```python
from build123d import *

# Parameters (mm, degrees)
ESQUISSE2_W             = 110
ESQUISSE2_H             = 106
BOSS_EXTRU_3_DEPTH      = 5
BOSS_EXTRU_4_DEPTH      = 3
BOSS_EXTRU_5_DEPTH      = 2
BOSS_EXTRU_6_DEPTH      = 5.5
BOSS_EXTRU_7_DEPTH      = 110
ESQUISSE7_R             = 2.35
ENL_V_MAT_EXTRU_1_DEPTH = 12
CONG_3_R                = 8
ENL_V_MAT_EXTRU_2_DEPTH = 4
CHANFREIN1_SIZE         = 0.5


with BuildPart() as part:
    # Esquisse2 → Boss.-Extru.3 (new body)
    with BuildSketch(Plane(origin=(0, 0, 0), x_dir=(1, 0, 0), z_dir=(0, 1, 0))):
        with Locations((55, 53)):
            Rectangle(ESQUISSE2_W, ESQUISSE2_H)
    extrude(amount=BOSS_EXTRU_3_DEPTH)

    # Esquisse3 → Boss.-Extru.4 (add)
    with BuildSketch(Plane(origin=(0, 5, 0), x_dir=(1, 0, 0), z_dir=(0, 1, 0))):
        Polygon((7, 4), (7, 106), (0, 106), (0, 0), (110, 0), (110, 106), (103, 106), (103, 4), align=None)
    extrude(amount=BOSS_EXTRU_4_DEPTH)

    # Esquisse4 → Boss.-Extru.5 (add)
    with BuildSketch(Plane(origin=(0, 8, 0), x_dir=(1, 0, 0), z_dir=(0, 1, 0))):
        Polygon((4, 106), (4, 4), (106, 4), (106, 106), (110, 106), (110, 0), (0, 0), (0, 106), align=None)
    extrude(amount=BOSS_EXTRU_5_DEPTH)

    # Esquisse6 → Boss.-Extru.6 (add)
    with BuildSketch(Plane(origin=(0, 10, 0), x_dir=(1, 0, 0), z_dir=(0, 1, 0))):
        Polygon((0, 106), (7, 106), (7, 4), (103, 4), (103, 106), (110, 106), (110, 4), (110, 0), (0, 0), (0, 4), align=None)
    extrude(amount=BOSS_EXTRU_6_DEPTH)

    # Esquisse8 → Boss.-Extru.7 (add)
    with BuildSketch(Plane(origin=(110, 0, 0), x_dir=(0, 0, -1), z_dir=(1, 0, 0))):
        Polygon((0, 0), (106, 0), (106, -18.690659955), align=None)
    extrude(amount=-BOSS_EXTRU_7_DEPTH)

    # Esquisse7 → Enlèv. mat.-Extru.1 (cut)
    with BuildSketch(Plane(origin=(0, 0, -106), x_dir=(-1, 0, 0), z_dir=(0, 0, -1))):
        with Locations((-103, 0)):
            Circle(ESQUISSE7_R)
        with Locations((-7, 0)):
            Circle(ESQUISSE7_R)
    extrude(amount=-ENL_V_MAT_EXTRU_1_DEPTH, mode=Mode.SUBTRACT)

    # Congé3
    cong_3_edges = [part.edges().sort_by_distance(p)[0] for p in [
        (110, 7.75, 0),
        (0, 7.75, 0),
    ]]
    fillet(cong_3_edges, radius=CONG_3_R)

    # Esquisse9 → Enlèv. mat.-Extru.2 (cut)
    with BuildSketch(Plane(origin=(0, 0, 0), x_dir=(1, 0, 0), z_dir=(0, -0.9848077530122092, 0.17364817766692348))):
        with BuildLine():
            Line((14, -8), (96, -8))
            ThreePointArc((96, -8), (100.242640687, -9.757359313), (102, -14))
            Line((102, -14), (102, -97.63522086))
            ThreePointArc((102, -97.63522086), (100.242640687, -101.877861547), (96, -103.63522086))
            Line((96, -103.63522086), (14, -103.63522086))
            ThreePointArc((14, -103.63522086), (9.757359313, -101.877861547), (8, -97.63522086))
            Line((8, -97.63522086), (8, -14))
            ThreePointArc((8, -14), (9.757359313, -9.757359313), (14, -8))
        make_face()
    extrude(amount=-ENL_V_MAT_EXTRU_2_DEPTH, mode=Mode.SUBTRACT)

    # Chanfrein1
    chanfrein1_edges = [part.edges().sort_by_distance(p)[0] for p in [
        (105.35, 0, -106),
        (9.35, 0, -106),
    ]]
    chamfer(chanfrein1_edges, length=CHANFREIN1_SIZE)


solid = part.part
```
Work out the finished part from the listing and answer in its coordinate system (mm). A direction names the side the tool comes from. Coordinates: 2 decimals unless noted, no trailing zeros. Order: outer loops, then holes, each group sorted by start corner. A loop starts at its lowest first (then second) coordinate and runs counter-clockwise, first axis right, second up. Notation, with made-up numbers: M 67.5,-28.75 L 111.5,-28.75 A19 cw 111.5,-21.75 Z; hole C 75,62.25 d4. An arc over 180 degrees is marked long. Use CSV: the item, a comma, the result in double quotes.
1) For faces 5 (the face through (7, 6, -54)), 6 (the face through (105, 10, -56)), 7 (the face through (100.2, 0.26, -9.91)), determine the directions among +Z, -Z, +X, -X, +Y, -Y from which every point of the face is accessible in a straight line to the end or side of a thin tool.
Worked out:
face 5,"-Z, +Y"
face 6,"-Z"
face 7,"-Y"
2) Section D-D on z = -98.5 is taken. Count the separate pieces of the cut face and the enclosed holes in it, plus the area to 3 significant figures.
Worked out:
separate pieces,"1"
enclosed holes,"2"
area,"2,180 mm^2"
3) Section B-B on z = -27.5 is taken. Write down the section's boundary in (x, y).
Worked out:
outline,"M 0,-4.85 L 8,-4.85 L 8,-0.79 L 102,-0.79 L 102,-4.85 L 110,-4.85 L 110,15.5 L 103,15.5 L 103,10 L 106,10 L 106,8 L 103,8 L 103,5 L 7,5 L 7,8 L 4,8 L 4,10 L 7,10 L 7,15.5 L 0,15.5 Z"
4) Flat-ended cylindrical pins translate along their axes: pin 1 Ø3 at (y, z) = (-10.5, -42) entering from +X; pin 2 Ø2.5 at (x, z) = (104.5, -57.5) entering from -Y; pin 3 Ø1.5 at (x, z) = (13, -66) entering from +Y; pin 4 Ø15 at (y, z) = (-12.5, -35) entering from +X. Find the tip coordinate at first contact, or state that the pin passes through.
Worked out:
pin 1,"passes through"
pin 2,"stops at y = -10.36"
pin 3,"stops at y = 5"
pin 4,"stops at x = 110"
5) Determine the mould class of faces 1 (the face through (55.257, -1.082, -6.136)), 2 (the face through (55.574, -16.054, -102.403)), 3 (the face through (107.719, 7.163, -2.406)), 4 (the face through (55, 15.5, -2)) for opening direction Y: released by +Y, released by -Y, zero draft, split by the parting line, or undercut.
Worked out:
face 1,"released by -Y"
face 2,"undercut"
face 3,"zero draft"
face 4,"released by +Y"
6) Section C-C on y = -6 is taken. Write down the section's boundary in (x, z).
Worked out:
outline,"M 0,-106 L 110,-106 L 110,-34.03 L 102,-34.03 L 102,-57.06 L 8,-57.06 L 8,-34.03 L 0,-34.03 Z"
7) Section A-A on x = 34 is taken. Write down the section's boundary in (y, z).
Worked out:
outline,"M -18.69,-106 L 5,-106 L 5,-4 L 15.5,-4 L 15.5,0 L 0,0 L -1.39,-7.88 L 2.55,-8.57 L -14.06,-102.76 L -18,-102.06 Z"
8) Consider line 1 (X direction, y = 9, z = -55.5); line 2 (X direction, y = 7, z = -71.5); line 3 (Z direction, x = 68.5, y = 7). Determine where each line is inside the solid, lowest interval first. Write a range as [from, to].
Worked out:
line 1,"x = [0, 4], [106, 110]"
line 2,"x = [0, 7], [103, 110]"
line 3,"z = [-4, 0]"
